For this review, take the finished solid that the model builds, in its own axes (mm). Face numbers are marked on the shaded views. A direction names the side the tool comes from. Round coordinates to 2 decimals unless told otherwise and drop trailing zeros. Write each loop counter-clockwise with the first axis right and the second up, starting at its lowest first coordinate (ties: lowest second). Pieces come first, ordered by that corner, then holes. Notation, with made-up numbers: (46, 43.25) -> (54, 43.25) arc R27 ccw to (54, 61.25) -> close; hole circle Ø6 at (-29, 19). An arc over 180 degrees is marked (long way). Answer as CSV lines item,"result". Start each with the question number.
Item 1: Take a section at A-A on z = 357. Give the boundary of the cut face in (x, y) (3 decimals).
Item 2: Take a section at B-B on x = -38.5. Give the boundary of the cut face in (y, z) (3 decimals).
Item 3: Wall thickness on probe 1 along Y at (x, z) = (-114, 279.5); probe 2 along Z at (x, y) = (-76, -1.25); probe 3 along Y at (x, z) = (-113, 330): over which ranges is each line inside the solid? List them lowest first. Write a range as from..to.
Item 4: For pin 1 Ø8 at (y, z) = (6, 335) entering from -X; pin 2 Ø2 at (y, z) = (2.5, 252) entering from +X; pin 3 Ø4 at (x, y) = (-49, 6) entering from +Z, all flat-tipped, find the tip position at first contact; note any pin that passes through.
Item 5: Machinability: for the marked faces 1, 2 and 3, which of the approach directions +Z, -Z, +X, -X, +Y, -Y give a long, thin tool a straight path to every point of the face, cutting with its end or side? Answer none if there is none.
Autodesk Inventor part; units mm, degrees
ref_plane "Work Plane1" through (0, 0, 203.2) normal (0, 0, 1) x (1, 0, 0)
ref_plane "YZ Plane" through (0, 0, 0) normal (1, 0, 0) x (0, 1, 0)
ref_plane "XZ Plane" through (0, 0, 0) normal (0, 1, 0) x (-1, 0, 0)
sketch "Sketch1" plane through (0, 0, 0) normal (0, 1, 0) x (-1, 0, 0)
  line L0 (0, 0) -> (0, 88.9)
  line L1 (12.7, 101.6) -> (101.6, 101.6)
  line L2 (114.3, 114.3) -> (114.3, 431.8)
  arc A0 (101.6, 101.6) -> (114.3, 114.3) centre (101.6, 114.3) ccw
  arc A1 (12.7, 101.6) -> (0, 88.9) centre (12.7, 88.9) ccw
  point P0 (0, 101.6)
  point P1 (114.3, 101.6)
  dimension "short" = 101.6
  dimension "right" = 114.3
  dimension "long" = 330.2
  dimension "turn_radius" = 12.7
  dimension "d10" = 12.7
sketch "Sketch2" plane through (0, 0, 0) normal (0, 0, 1) x (1, 0, 0)
  circle A0 centre (0, 0) radius 12.7
  circle A1 centre (0, 0) radius 9.525
  dimension "outsideDiam" = 25.4
  dimension "insideDiam" = 19.05
sweep "Sweep2" add profiles "Sketch2" path "Sketch1"
ref_plane "Work Plane1" through (0, 0, 203.2) normal (0, 0, 1) x (1, 0, 0)
properties part number "AsBuilt Aluminum Arm" material "Aluminum 6061"
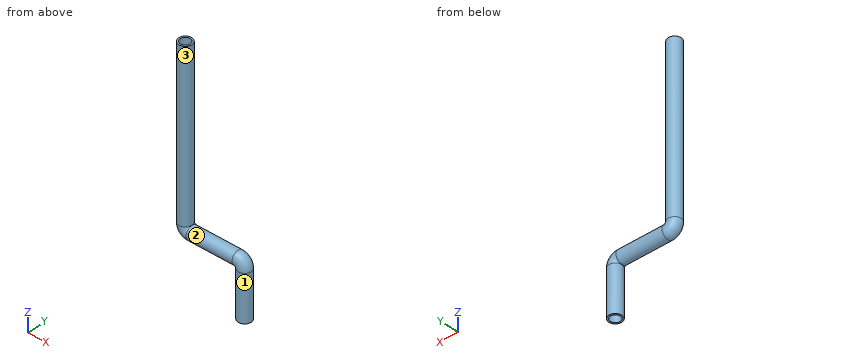
Output values:
1,outline,"circle Ø25.4 at (-114.3, 0); hole circle Ø19.05 at (-114.3, 0)"
2,outline,"circle Ø25.4 at (0, 101.6); hole circle Ø19.05 at (0, 101.6)"
3,probe 1,"y = -12.7..-9.52, 9.52..12.7"
3,probe 2,"z = 88.96..92.16, 111.04..114.24"
3,probe 3,"y = -12.63..-9.44, 9.44..12.63"
4,pin 1,"stops at x = -126.84"
4,pin 2,"stops at x = -101.69"
4,pin 3,"stops at z = 113.65"
5,face 1,"-Z"
5,face 2,"none"
5,face 3,"+Z"
